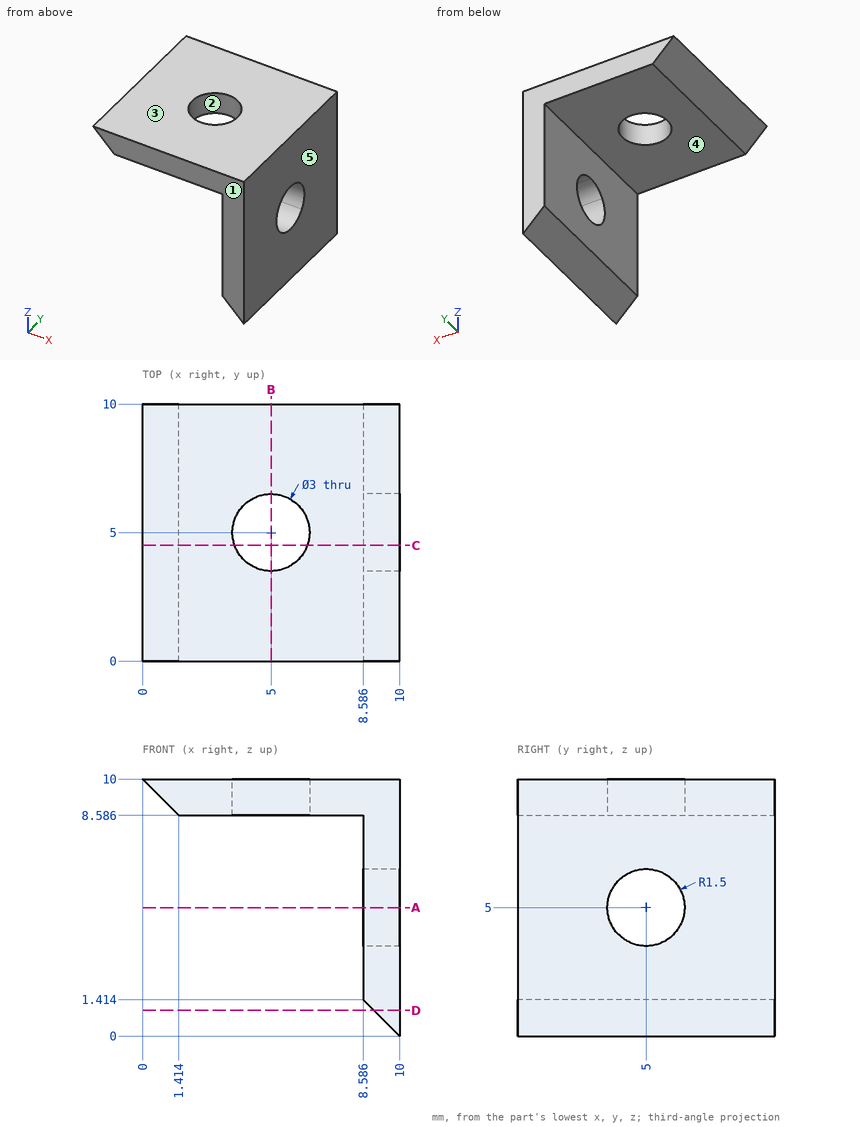
The drawing under review shows one solid part. Ordinate dimensions are in mm from its lowest x, y, z. A direction names the side the tool comes from. Coordinates: 2 decimals unless noted, no trailing zeros. Write each loop counter-clockwise with the first axis right and the second up, starting at its lowest first coordinate (ties: lowest second). Pieces come first, ordered by that corner, then holes. Notation, with made-up numbers: M 39,55.25 L 80,55.25 A18 cw 80,64.25 Z; hole C 69,-14 d11. An arc over 180 degrees is marked long. Answer as a JSON object with one key per item and string values.
Item 1: Add section C-C, the plane y = 4.5. Give the boundary of the cut face in (x, z).
Outcome:
{"outline": "M 0,10 L 1.41,8.59 L 3.59,8.59 L 3.59,10 Z; M 6.41,8.59 L 8.59,8.59 L 8.59,6.41 L 10,6.41 L 10,10 L 6.41,10 Z; M 8.59,1.41 L 10,0 L 10,3.59 L 8.59,3.59 Z"}
Item 2: Add section B-B, the plane x = 5. Give the boundary of the cut face in (y, z).
Outcome:
{"outline": "M 0,8.59 L 3.5,8.59 L 3.5,10 L 0,10 Z; M 6.5,8.59 L 10,8.59 L 10,10 L 6.5,10 Z"}
Item 3: Insertion check: pin 1 Ø1 at (y, z) = (7.5, 8.5) entering from -X; pin 2 Ø3 at (x, y) = (4.5, 3) entering from -Z; pin 3 Ø5.5 at (y, z) = (5, 5.5) entering from -X. Each pin has a flat end and moves straight along its axis. Give the tip position at first contact, or say it passes through.
Outcome:
{"pin 1": "x = 1", "pin 2": "z = 8.59", "pin 3": "x = 8.59"}
Item 4: Draft analysis for pull direction Y (two halves, no side actions). For the marked faces 1, 2 and 3, state which applies: pulls with the +Y half, pulls with the -Y half, needs draft (parallel to the pull), parting line crosses it, or undercut.
Outcome:
{"face 1": "pulls with the -Y half", "face 2": "undercut", "face 3": "needs draft"}
Item 5: Add section D-D, the plane z = 1. Give the boundary of the cut face in (x, y), and give its area (3 significant figures).
Outcome:
{"outline": "M 9,0 L 10,0 L 10,10 L 9,10 Z", "area": "10.0 mm²"}
Item 6: Wall thickness on probe 1 along Z at (x, y) = (5.25, 9); probe 2 along Y at (x, z) = (5, 9.75): over which ranges is each line inside the solid? List them lowest first.
Outcome:
{"probe 1": "8.59 to 10", "probe 2": "0 to 3.5, 6.5 to 10"}
Item 7: Add section A-A, the plane z = 5. Give the boundary of the cut face in (x, y).
Outcome:
{"outline": "M 8.59,0 L 10,0 L 10,3.5 L 8.59,3.5 Z; M 8.59,6.5 L 10,6.5 L 10,10 L 8.59,10 Z"}
Item 8: Machinability: for the marked faces 4 and 5, which of the approach directions +Z, -Z, +X, -X, +Y, -Y give a long, thin tool a straight path to every point of the face, cutting with its end or side? Answer none if there is none.
Outcome:
{"face 4": "-Z, -X, +Y, -Y", "face 5": "+Z, -Z, +X, +Y, -Y"}
